Check sheet for the modelled part. Datum: model origin and axes. Units: mm. Face numbers are marked on the shaded views. A direction names the side the tool comes from. Give positions to 0.01 mm unless a question says otherwise; leave off trailing zeros. Order: outer loops, then holes, each group sorted by start corner. A loop starts at its lowest first (then second) coordinate and runs counter-clockwise, first axis right, second up.
Item 1: Access from +Z, -Z, +X, -X, +Y, -Y to the whole of each face (thin tool, end or side, straight path). Record for the marked faces 1 and 2.
Item 2: Material ranges on line 1 along X through (y, z) = (12, 10.5); line 2 along Z through (x, y) = (63.5, 22.5); line 3 along Y through (x, z) = (45.5, 5), recorded low to high.
Item 3: Release check for a two-part mould opening along X. For the marked faces 3, 4, 5 and 6 record: released by +X, released by -X, zero draft, split by the parting line, or undercut.
Item 4: Gauge pin test, flat ends, axial feed: P1, Ø12, axis at x = 43, y = 17, coming from the -Z side; P2, Ø5, axis at x = 51, z = 7, coming from the +Y side; P3, Ø6, axis at x = 56.5, y = 12, coming from the +Z side. Record the tip position at first contact, or that the pin passes through.
Item 5: Sectioned sample at B-B on y = 21.5. Record the boundary of the cut face in (x, z).
Item 6: Sectioned sample at A-A on z = 4. Record the boundary of the cut face in (x, y).
Item 7: Sectioned sample at C-C on x = 10.5. Record the boundary of the cut face in (y, z).
from build123d import *

# Parameters (mm, degrees)
F0_W     = 69.2
F0_H     = 32
F1_DEPTH = 2
F3_DEPTH = 9.5
F4_W     = 66.2
F4_H     = 1.5
F5_DEPTH = 9.5


with BuildPart() as f1:
    # F0 (on Top) → F1 (new body)
    with BuildSketch(Plane.XY):
        with Locations((34.6, 16)):
            Rectangle(F0_W, F0_H)
    extrude(amount=F1_DEPTH)

    # F2 (on face) → F3 (join)
    with BuildSketch(Plane.XY.offset(2)):
        Polygon((3.5, 32), (0, 32), (0, 0), (69.2, 0), (69.2, 32), (65.7, 32), (65.7, 30.5), (67.7, 30.5), (67.7, 1.5), (1.5, 1.5), (1.5, 30.5), (3.5, 30.5), align=None)
    extrude(amount=F3_DEPTH)

    # F4 (on face) → F5 (cut)
    with BuildSketch(Plane.XY.offset(11.5)):
        with Locations((34.6, 31.25)):
            Rectangle(F4_W, F4_H)
    extrude(amount=-F5_DEPTH, mode=Mode.SUBTRACT)


solid = f1.part
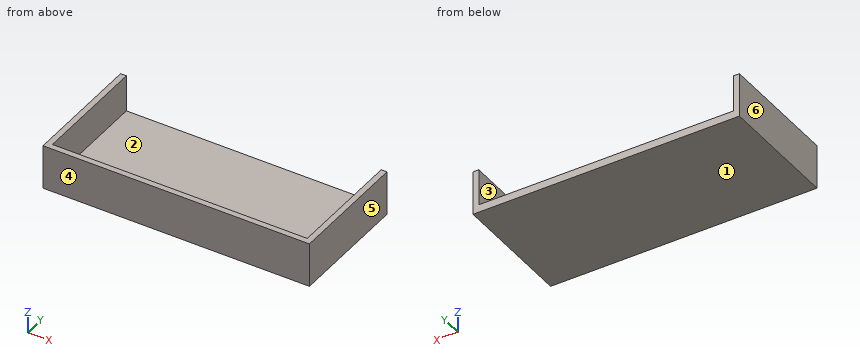
Report:
1. face 1: -Z, +X, -X, +Y, -Y
1. face 2: +Z, +Y
2. line 1: x = 0 to 1.5, 67.7 to 69.2
2. line 2: z = 0 to 2
2. line 3: y = 0 to 1.5
3. face 3: undercut
3. face 4: zero draft
3. face 5: released by +X
3. face 6: released by -X
4. P1: stops at z = 0
4. P2: stops at y = 1.5
4. P3: stops at z = 2
5. outline: (0, 0) - (69.2, 0) - (69.2, 11.5) - (67.7, 11.5) - (67.7, 2) - (1.5, 2) - (1.5, 11.5) - (0, 11.5) - close
6. outline: (0, 0) - (69.2, 0) - (69.2, 32) - (67.7, 32) - (67.7, 1.5) - (1.5, 1.5) - (1.5, 32) - (0, 32) - close
7. outline: (0, 0) - (32, 0) - (32, 2) - (1.5, 2) - (1.5, 11.5) - (0, 11.5) - close
